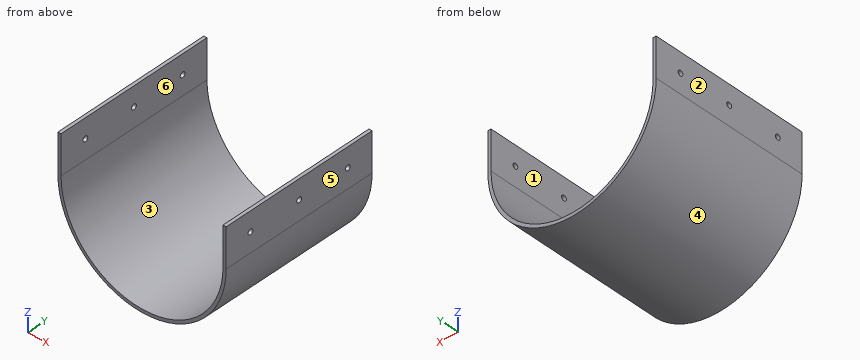
from build123d import *

# Parameters (mm, degrees)
BOSS_EXTRUDE1_DEPTH = 150
SKETCH2_R           = 2.5
CUT_EXTRUDE1_DEPTH  = 161


with BuildPart() as part:
    # Sketch1 → Boss-Extrude1 (new body)
    with BuildSketch(Plane(origin=(0, 0, 0), x_dir=(1, 0, 0), z_dir=(0, 1, 0))):
        with BuildLine():
            Line((-80.885057471, 0), (-80.885057471, -37.067376772))
            Line((-80.885057471, -37.067376772), (-77.885057471, -37.067376772))
            Line((-77.885057471, -37.067376772), (-77.885057471, 0))
            ThreePointArc((-77.885057471, 0), (-0.885057471, 77), (76.114942529, 0))
            Line((76.114942529, 0), (76.114942529, -37.067376772))
            Line((76.114942529, -37.067376772), (79.114942529, -37.067376772))
            Line((79.114942529, -37.067376772), (79.114942529, 0))
            ThreePointArc((79.114942529, 0), (-0.885057471, 80), (-80.885057471, 0))
        make_face()
    extrude(amount=BOSS_EXTRUDE1_DEPTH)

    # Sketch2 → Cut-Extrude1 (cut, through all)
    with BuildSketch(Plane(origin=(79.114942529, 0, 0), x_dir=(0, 0, -1), z_dir=(1, 0, 0))):
        with Locations((-18.5, 125)):
            Circle(SKETCH2_R)
        with Locations((-18.5, 75)):
            Circle(SKETCH2_R)
        with Locations((-18.5, 25)):
            Circle(SKETCH2_R)
    extrude(amount=-CUT_EXTRUDE1_DEPTH, mode=Mode.SUBTRACT)


solid = part.part
For this review, take the finished solid that the model builds, in its own axes (mm). Face numbers are marked on the shaded views. A direction names the side the tool comes from. Round coordinates to 2 decimals unless told otherwise and drop trailing zeros. Order: outer loops, then holes, each group sorted by start corner. A loop starts at its lowest first (then second) coordinate and runs counter-clockwise, first axis right, second up. Notation, with made-up numbers: M 5.25,84.5 L 13.25,84.5 A21 cw 13.25,106.5 Z; hole C 18.25,-22.5 d2. An arc over 180 degrees is marked long. Use a Markdown table: item, result. Add a question column.
Item 1: Tool access review of the marked faces 1 and 2: name each direction out of +Z, -Z, +X, -X, +Y, -Y from which nothing blocks a thin tool from reaching the whole face with its end or side.
Item 2: To check wall thickness, follow line 1 along Y through (x, z) = (-80, 18); line 2 along Y through (x, z) = (77.65, 18.5); line 3 along X through (y, z) = (72.5, 23). State the ranges of each line that lie inside material, in increasing order.
Item 3: Add section D-D, the plane z = -34.5. Give the boundary of the cut face in (x, y), then the cut area to 3 significant figures.
Item 4: Insertion check: pin 1 (10 mm diameter, centred on x = -2, y = 22, fed in from +Z); pin 2 (1.5 mm diameter, centred on x = -60, y = 61, fed in from -Z); pin 3 (6 mm diameter, centred on x = -64.5, y = 105.5, fed in from +Z). Each pin has a flat end and moves straight along its axis. Give the tip position at first contact, or say it passes through.
Item 5: Add section C-C, the plane y = 42.5. Give the boundary of the cut face in (x, z), then the cut area to 3 significant figures.
Item 6: Add section A-A, the plane y = 125. Give the boundary of the cut face in (x, z).
Item 7: Add section B-B, the plane z = 29. Give the boundary of the cut face in (x, y), then the cut area to 3 significant figures.
Item 8: Mouldability with a two-part tool opening along X and no side actions: class the marked faces 3, 4, 5 and 6 as released by +X, released by -X, zero draft, split by the parting line, or undercut.
Geometry results:
| question | item | result |
|---|---|---|
| 1 | face 1 | +Z, +Y, -Y |
| 1 | face 2 | +Z, -Z, -X, +Y, -Y |
| 2 | line 1 | y = 0 to 22.55, 27.45 to 72.55, 77.45 to 122.55, 127.45 to 150 |
| 2 | line 2 | y = 0 to 22.5, 27.5 to 72.5, 77.5 to 122.5, 127.5 to 150 |
| 2 | line 3 | x = -80.89 to -77.89, 76.11 to 79.11 |
| 3 | outline | M -73.06,0 L -69.72,0 L -69.72,150 L -73.06,150 Z; M 67.95,0 L 71.29,0 L 71.29,150 L 67.95,150 Z |
| 3 | area | 1,000 mm² |
| 4 | pin 1 | stops at z = -76.76 |
| 4 | pin 2 | stops at z = -54.71 |
| 4 | pin 3 | stops at z = -38.62 |
| 5 | outline | M -80.89,0 A80 ccw 79.11,0 L 79.11,37.07 L 76.11,37.07 L 76.11,0 A77 cw -77.89,0 L -77.89,37.07 L -80.89,37.07 Z |
| 5 | area | 962 mm² |
| 6 | outline | M -80.89,0 A80 ccw 79.11,0 L 79.11,16 L 76.11,16 L 76.11,0 A77 cw -77.89,0 L -77.89,16 L -80.89,16 Z; M -80.89,21 L -77.89,21 L -77.89,37.07 L -80.89,37.07 Z; M 76.11,21 L 79.11,21 L 79.11,37.07 L 76.11,37.07 Z |
| 7 | outline | M -80.89,0 L -77.89,0 L -77.89,150 L -80.89,150 Z; M 76.11,0 L 79.11,0 L 79.11,150 L 76.11,150 Z |
| 7 | area | 900 mm² |
| 8 | face 3 | undercut |
| 8 | face 4 | split by the parting line |
| 8 | face 5 | released by +X |
| 8 | face 6 | undercut |
